Design review of the part built by this model. Coordinates are the model's own, in mm. A direction names the side the tool comes from. Give positions to 0.01 mm unless a question says otherwise; leave off trailing zeros. Loops run counter-clockwise (first coordinate to the right, second up) from the corner with the lowest first, then second, coordinate; pieces in that order, holes last. Notation, with made-up numbers: M -26.75,83.5 L 27.25,83.5 A18 cw 27.25,100.5 Z; hole C 41.25,37.25 d3. An arc over 180 degrees is marked long. Use one line per item in the form item = value. Start each with the question number.
from build123d import *

# Parameters (mm, degrees)
F2_R = 50.8
F0_R = 38.1
F5_T = -5.08


with BuildPart() as f3:
    # F2 (on offset) → F3 section 0
    with BuildSketch(Plane.XY.offset(50.8)):
        Circle(F2_R)
    # F0 (on Top) → F3 section 1
    with BuildSketch(Plane.XY):
        Circle(F0_R)
    loft()

    # F4: F3 across plane


with BuildPart() as f3_1:
    add(f3.part)
    add(f3.part.mirror(Plane.XY))

    # F5
    f5_openings = [f3_1.faces().sort_by_distance(p)[0] for p in [
        (0, 0, -50.8),
        (0, 0, 50.8),
    ]]
    offset(amount=F5_T, openings=f5_openings, kind=Kind.INTERSECTION)


solid = f3_1.part
Q1. Take a section at A-A on x = 0. Give the boundary of the cut face in (y, z), plus the area to 3 significant figures.
Q2. Wall thickness on probe 1 along Y at (x, z) = (-25, 2.5); probe 2 along X at (y, z) = (12.5, -46); probe 3 along X at (y, z) = (17.5, 33): over which ranges is each line inside the solid? List them lowest first.
Q3. Take a section at B-B on z = 27. Give the boundary of the cut face in (x, y).
Q4. Take a section at C-C on z = -13.5. Give the boundary of the cut face in (x, y) (3 decimals), plus the area to 3 significant figures.
Q5. For faces 1 (the flat face through (-19, 42, 50.8)), 2 (the conical face through (-41.5, 1.83, -13.76)), list the 3-axis set-ups (+Z, -Z, +X, -X, +Y, -Y) from which the entire face can be reached by the end or side of a thin tool; tool diameter is ignored.
Q6. The part is to be moulded in two halves that separate along Y. For faces 3 (the conical face through (33.534, -13.904, -13.756)), 4 (the conical face through (-41.5, 1.83, 13.76)), 5 (the flat face through (-19, 42, -50.8)), say which applies: pulls with the +Y half, pulls with the -Y half, needs draft (parallel to the pull), parting line crosses it, or undercut.
Q7. Clearance check with flat-ended pins moving along their axes: pin 1 Ø1 at (y, z) = (24.5, 21.5) entering from +X; pin 2 Ø6 at (y, z) = (32.5, -11) entering from +X; pin 3 Ø10 at (y, z) = (-32.5, -28.5) entering from +X. State where each tip first meets the part, or that it passes through.
Response values:
q1.outline = M -50.8,-50.8 L -45.56,-50.8 L -32.86,0 L -45.56,50.8 L -50.8,50.8 L -38.1,0 Z; M 32.86,0 L 45.56,-50.8 L 50.8,-50.8 L 38.1,0 L 50.8,50.8 L 45.56,50.8 Z
q1.area = 1,060 mm^2
q2.probe_1 = -29.57 to -22.28, 22.28 to 29.57
q2.probe_2 = -48 to -42.57, 42.57 to 48
q2.probe_3 = -42.92 to -37.2, 37.2 to 42.92
q3.outline = C 0,0 d89.7; hole C 0,0 d79.23
q4.outline = C 0,0 d82.95; hole C 0,0 d72.477
q4.area = 1,280 mm^2
q5.face_1 = +Z, +X, -X, +Y, -Y
q5.face_2 = none
q6.face_3 = undercut
q6.face_4 = parting line crosses it
q6.face_5 = needs draft
q7.pin_1 = 36.28
q7.pin_2 = 28.44
q7.pin_3 = 36.21
